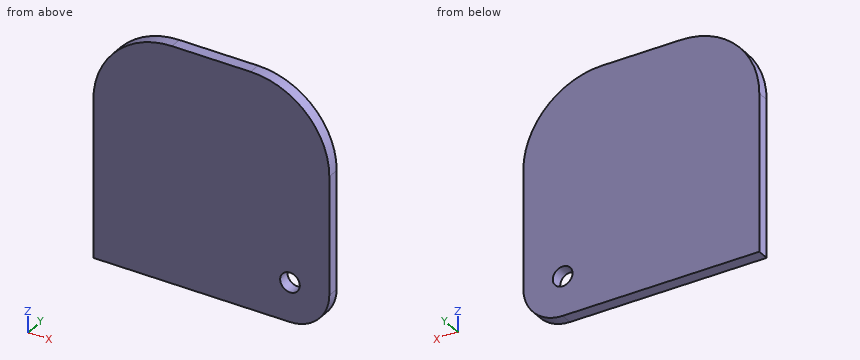
Autodesk Inventor part; units mm, degrees
ref_plane "YZ Plane" through (0, 0, 0) normal (1, 0, 0) x (0, 1, 0)
ref_plane "XZ Plane" through (0, 0, 0) normal (0, 1, 0) x (-1, 0, 0)
ref_plane "XY Plane" through (0, 0, 0) normal (0, 0, 1) x (1, 0, 0)
sketch "Sketch1" plane through (0, 0, 0) normal (0, 1, 0) x (-1, 0, 0)
  line L0 (0, 0) -> (76.2, 0)
  line L1 (76.2, 0) -> (76.2, 76.2)
  line L2 (76.2, 76.2) -> (0, 76.2)
  line L3 (0, 76.2) -> (0, 0)
  dimension "d0" = 76.2
  dimension "d1" = 76.2
extrude "Extrusion1" add sketch "Sketch1" along normal blind 3.81
sketch "Sketch2" plane through (0, 3.81, 0) normal (0, 1, 0) x (1, 0, 0)
  circle A0 centre (-12.7, -12.7) radius 12.7
  circle A1 centre (-12.7, -12.7) radius 3.175
  line L0 (0, 0) -> (-76.2, 0)
  line L1 (0, -76.2) -> (0, 0)
  dimension "d4" = 25.4
extrude "Extrusion2" cut sketch "Sketch2" against normal blind 3.81 contours A1
sketch "Sketch3" plane through (0, 0, 0) normal (0, -1, 0) x (1, 0, 0)
  circle A0 centre (-12.7, 12.7) radius 3.175
  circle A1 centre (-12.7, 12.7) radius 12.7
  line L0 (0, 76.2) -> (0, 0)
  line L1 (0, 0) -> (-76.2, 0)
  line L2 (-12.7, 0) -> (0, 0)
  line L3 (0, 0) -> (0, 12.7)
extrude "Extrusion3" cut sketch "Sketch3" against normal blind 3.81 contours L0 L1 A1
fillet "Fillet1" radius 25.4 2 edges at (-76.2, 1.905, 76.2) (0, 1.905, 76.2)
properties part number "moving plate"
For this review, take the finished solid that the model builds, in its own axes (mm). Coordinates: 2 decimals unless noted, no trailing zeros. Write each loop counter-clockwise with the first axis right and the second up, starting at its lowest first coordinate (ties: lowest second). Pieces come first, ordered by that corner, then holes.
(1) Add section A-A on y = 1.8. Give the boundary of the cut face in (x, z) (3 decimals), then the cut area to 3 significant figures.
(2) Add section B-B on x = -69.5. Give the boundary of the cut face in (y, z).
(3) For pin 1 Ø5 at (x, z) = (-12.7, 12.7) entering from +Y, flat-tipped, find the tip position at first contact; note if it passes through.
(4) Wall thickness on probe 1 along X at (y, z) = (2.9, 12.7) (3 decimals); probe 2 along Z at (x, y) = (-12.7, 2.95) (3 decimals); probe 3 along Z at (x, y) = (-51.5, 1.1): over which ranges is each line inside the solid? List them lowest first.
Answer sheet:
1. outline: (-76.2, 0) - (-12.7, 0) arc R12.7 ccw to (0, 12.7) - (0, 50.8) arc R25.4 ccw to (-25.4, 76.2) - (-50.8, 76.2) arc R25.4 ccw to (-76.2, 50.8) - close; hole circle Ø6.35 at (-12.7, 12.7)
1. area: 5,460 mm2
2. outline: (0, 0) - (3.81, 0) - (3.81, 67.99) - (0, 67.99) - close
3. pin 1: passes through
4. probe 1: x = -76.2 to -15.875, -9.525 to 0
4. probe 2: z = 0 to 9.525, 15.875 to 72.797
4. probe 3: z = 0 to 76.19
